```python
from build123d import *

# Parameters (mm, degrees)
F0_W     = 546.8174844539
F0_H     = 398.7210936817
F1_DEPTH = 25.4
F3_DEPTH = 25.401
F4_R     = 5.08
F5_R     = 2.159


# Not quite as in the source:
# - a feature names something its author has since deleted; it is built from what else it names


with BuildPart() as f1:
    # F0 (on Front) → F1 (new body)
    with BuildSketch(Plane.XZ):
        with Locations((480.6314062452, -83.1606246494)):
            Rectangle(F0_W, F0_H)
        Polygon((330.755193297, 46.4165987058), (352.6924322393, 58.7807495217), (497.1109463772, 58.7807495217), (525.0629135844, 52.5692068872), (560.0028810439, 52.5692068872), (579.4140003676, 37.8167783416), (597.2722044557, 30.8287886525), (597.2722044557, 19.9585742536), (579.4140003676, 12.9705761138), (562.3322031939, 0), (493.2287427939, -14.9813921496), (476.9234201392, -48.3684665562), (464.5003348701, -54.5800176413), (451.3007750821, -98.8373032779), (493.3564558907, -111.380243164), (493.3564558907, -127.5657196522), (483.1349796749, -150.8590341088), (393.7753742012, -153.3092504783), (393.5303500451, -144.3731980569), (384.284519278, -144.626716252), (383.8496065952, -128.7654126401), (394.4104195536, -108.2215374956), (394.4104195536, -64.4587469067), (400.6219790893, -38.8361145254), (368.0113337798, -22.5307876454), (337.8036322085, -13.9719399936), (330.755193297, 21.270351746), align=None, mode=Mode.SUBTRACT)
    extrude(amount=F1_DEPTH)

    # F2 (on face) → F3 (cut, through all)
    with BuildSketch(Plane.XZ.offset(25.4)):
        Polygon((527.7804729939, -7.4906960748), (337.8036322085, -13.9719399936), (365.5445277691, -75.1346200705), (401.7401635647, -93.1630060077), (472.3286154864, -105.1087732209), align=None)
    extrude(amount=-F3_DEPTH, mode=Mode.SUBTRACT)

    # F4
    f4_edges = [f1.edges().sort_by_distance(p)[0] for p in [
        (330.755193, -12.7, 21.270352),
        (330.755193, -12.7, 46.416599),
        (352.692432, -12.7, 58.78075),
        (337.803632, -12.7, -13.97194),
        (394.41042, -12.7, -108.221537),
        (383.849607, -12.7, -128.765413),
        (384.284519, -12.7, -144.626716),
        (483.13498, -12.7, -150.859034),
        (493.356456, -12.7, -127.56572),
        (562.332203, -12.7, 0),
        (579.414, -12.7, 12.970576),
        (597.272204, -12.7, 19.958574),
        (493.356456, -12.7, -111.380243),
        (525.062914, -12.7, 52.569207),
        (560.002881, -12.7, 52.569207),
        (579.414, -12.7, 37.816778),
        (597.272204, -12.7, 30.828789),
        (497.110946, -12.7, 58.78075),
        (365.544528, -12.7, -75.13462),
        (472.328615, -12.7, -105.108773),
        (394.41042, -12.7, -89.512194),
        (527.780473, -12.7, -7.490696),
    ]]
    fillet(f4_edges, radius=F4_R)

    # F5
    f5_edges = [f1.edges().sort_by_distance(p)[0] for p in [
        (393.775374, -12.7, -153.30925),
    ]]
    fillet(f5_edges, radius=F5_R)


solid = f1.part
```
Can you work these out from the model? Positions are in its coordinate system, mm. A direction names the side the tool comes from. Round coordinates to 2 decimals unless told otherwise and drop trailing zeros. Loops run counter-clockwise (first coordinate to the right, second up) from the corner with the lowest first, then second, coordinate; pieces in that order, holes last.
Item 1: Suppose I cut it at A-A, the plane x = 588.5. Write out the boundary of the cut face in (y, z), then the cut area to 3 significant figures.
Item 2: Suppose I cut it at B-B, the plane z = -41. Write out the boundary of the cut face in (x, y), then the cut area to 3 significant figures.
Item 3: Which directions (+Z, -Z, +X, -X, +Y, -Y) give clear straight access to the entire face, cutting with the end or side of a thin tool? Please do faces 4 (the flat face through (351.234, -12.878, -43.584)), 5 (the flat face through (477, -13, -282.521)).
Item 4: Please list where these lines run through material, in increasing order: L1, parallel to Z at x = 590.5, y = -6; L2, parallel to Z at x = 575.5, y = -23.25; L3, parallel to X at y = -20.25, z = -112.
Item 5: If we mould it in two halves opening along X, with no side actions, what happens to faces 1 (the flat face through (569.99, -12.52, 44.98)), 2 (the flat face through (754.04, -13, -86)), 3 (the flat face through (207.223, -13, -86))? For each: +X half, -X half, draft (parallel to the pull), parting line (faces both ways), or undercut.
Reported:
1. outline: (-25.4, -282.52) - (0, -282.52) - (0, 16.53) - (-25.4, 16.53) - close; (-25.4, 34.26) - (0, 34.26) - (0, 116.2) - (-25.4, 116.2) - close
1. area: 9,680 mm2
2. outline: (207.22, -25.4) - (350.06, -25.4) - (350.06, 0) - (207.22, 0) - close; (508.75, -25.4) - (754.04, -25.4) - (754.04, 0) - (508.75, 0) - close
2. area: 9,860 mm2
3. face 4: +Y, -Y
3. face 5: -Z, +X, -X, +Y, -Y
4. L1: z = -282.52 to 17.31, 33.48 to 116.2
4. L2: z = -282.52 to 10, 40.79 to 116.2
4. L3: x = 207.22 to 392.47, 492.25 to 754.04
5. face 1: undercut
5. face 2: +X half
5. face 3: -X half
